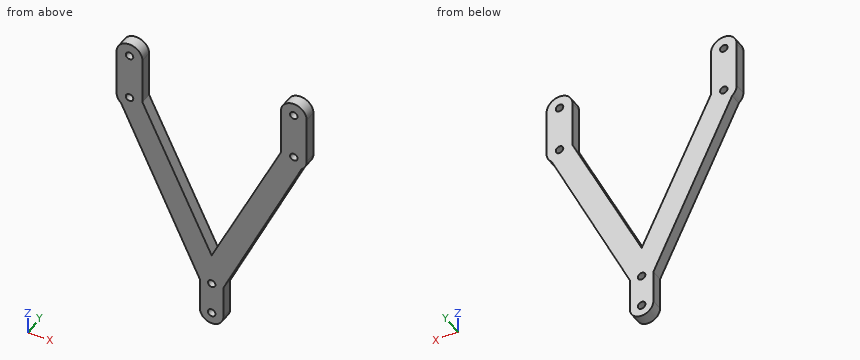
from build123d import *

# Parameters (mm, degrees)
SKETCH_1_R      = 1.6
SKETCH_1_R_2    = 1.634753067
EXTRUDE_1_DEPTH = 5


with BuildPart() as part:
    # 草图1 → 凸台-拉伸1 (new body)
    with BuildSketch(Plane(origin=(0, 0, 0), x_dir=(1, 0, 0), z_dir=(0, 1, 0))):
        with BuildLine():
            Line((-29.5, 11.78850637), (-29.5, -8.21149363))
            ThreePointArc((-29.5, -8.21149363), (-35, -13.71149363), (-40.5, -8.21149363))
            Line((-40.5, -8.21149363), (-40.5, 11.78850637))
            ThreePointArc((-40.5, 11.78850637), (-39.989553993, 14.102453419), (-38.552963292, 15.986893184))
            Line((-38.552963292, 15.986893184), (-5, 86.78850637))
            Line((-5, 86.78850637), (-5, 100.78850637))
            ThreePointArc((-5, 100.78850637), (0, 105.78850637), (5, 100.78850637))
            Line((5, 100.78850637), (5, 86.78850637))
            Line((5, 86.78850637), (38.348099221, 16.152017755))
            ThreePointArc((38.348099221, 16.152017755), (39.932775371, 14.221144268), (40.5, 11.78850637))
            Line((40.5, 11.78850637), (40.5, -8.21149363))
            ThreePointArc((40.5, -8.21149363), (35, -13.71149363), (29.5, -8.21149363))
            Line((29.5, -8.21149363), (29.5, 11.78850637))
            Line((29.5, 11.78850637), (0, 73.28850637))
            Line((0, 73.28850637), (-29.5, 11.78850637))
        make_face()
        with Locations((-35, -8.21149363)):
            Circle(SKETCH_1_R, mode=Mode.SUBTRACT)
        with Locations((-35, 11.78850637)):
            Circle(SKETCH_1_R, mode=Mode.SUBTRACT)
        with Locations((35, 11.78850637)):
            Circle(SKETCH_1_R, mode=Mode.SUBTRACT)
        with Locations((35, -8.21149363)):
            Circle(SKETCH_1_R, mode=Mode.SUBTRACT)
        with Locations((0, 100.78850637)):
            Circle(SKETCH_1_R_2, mode=Mode.SUBTRACT)
        with Locations((0, 86.78850637)):
            Circle(SKETCH_1_R, mode=Mode.SUBTRACT)
    extrude(amount=EXTRUDE_1_DEPTH)


solid = part.part
Input: part model. Units: mm. Frame: model coordinates. Coordinates: 2 decimals unless noted, no trailing zeros. Order: outer loops, then holes, each group sorted by start corner. A loop starts at its lowest first (then second) coordinate and runs counter-clockwise, first axis right, second up. Notation, with made-up numbers: M 26,-36.75 L 84,-36.75 A15 cw 84,-14.75 Z; hole C 18.25,60.5 d9. An arc over 180 degrees is marked long. Answer in a Markdown table with one row per item.
(1) Section query A-A, the plane z = 0. Output: boundary loops of the cut face in (x, y).
Numbers:
| item | result |
|---|---|
| outline | M -40.5,0 L -29.5,0 L -29.5,5 L -40.5,5 Z; M 29.5,0 L 40.5,0 L 40.5,5 L 29.5,5 Z |
(2) Material intervals for line 1 (X direction, y = 4.8, z = 8); line 2 (X direction, y = 2.25, z = 6); line 3 (Z direction, x = 35, y = 1.6), sorted ascending. Write a range as [from, to].
Numbers:
| item | result |
|---|---|
| line 1 | x = [-40.5, -36.59], [-33.41, -29.5], [29.5, 33.41], [36.59, 40.5] |
| line 2 | x = [-40.5, -29.5], [29.5, 40.5] |
| line 3 | z = [-23.24, -13.39], [-10.19, 6.61], [9.81, 13.71] |
(3) Section query D-D, the plane z = -42. Output: boundary loops of the cut face in (x, y).
Numbers:
| item | result |
|---|---|
| outline | M -26.23,0 L -15.01,0 L -15.01,5 L -26.23,5 Z; M 15.01,0 L 26.15,0 L 26.15,5 L 15.01,5 Z |
(4) Contact query for flat-ended pins moving along their axis: pin 1 Ø1.5 at (y, z) = (2, -95) entering from +X; pin 2 Ø1 at (x, y) = (-9.5, 1) entering from +Z; pin 3 Ø1 at (x, y) = (29, 3) entering from -Z. Output: stop coordinate, or through.
Numbers:
| item | result |
|---|---|
| pin 1 | stops at x = 5 |
| pin 2 | stops at z = -52.44 |
| pin 3 | stops at z = -37.01 |
(5) Section query C-C, the plane x = -35. Output: boundary loops of the cut face in (y, z), plus the area to 3 significant figures.
Numbers:
| item | result |
|---|---|
| outline | M 0,-23.48 L 5,-23.48 L 5,-13.39 L 0,-13.39 Z; M 0,-10.19 L 5,-10.19 L 5,6.61 L 0,6.61 Z; M 0,9.81 L 5,9.81 L 5,13.71 L 0,13.71 Z |
| area | 154 mm^2 |
(6) Section query B-B, the plane y = 2.85. Output: boundary loops of the cut face in (x, z), plus the area to 3 significant figures.
Numbers:
| item | result |
|---|---|
| outline | M -40.5,-11.79 A5.5 ccw -38.55,-15.99 L -5,-86.79 L -5,-100.79 A5 ccw 5,-100.79 L 5,-86.79 L 38.35,-16.15 A5.5 ccw 40.5,-11.79 L 40.5,8.21 A5.5 ccw 29.5,8.21 L 29.5,-11.79 L 0,-73.29 L -29.5,-11.79 L -29.5,8.21 A5.5 ccw -40.5,8.21 Z; hole C -35,-11.79 d3.2; hole C -35,8.21 d3.2; hole C 0,-100.79 d3.27; hole C 0,-86.79 d3.2; hole C 35,-11.79 d3.2; hole C 35,8.21 d3.2 |
| area | 2,270 mm^2 |
